Design review of the part built by this model. Coordinates are the model's own, in mm. Face numbers are marked on the shaded views. A direction names the side the tool comes from. Coordinates: 2 decimals unless noted, no trailing zeros. Write each loop counter-clockwise with the first axis right and the second up, starting at its lowest first coordinate (ties: lowest second). Pieces come first, ordered by that corner, then holes. Notation, with made-up numbers: (1, -13) -> (29, -13) arc R18 cw to (29, -7) -> close; hole circle Ø8 at (15.5, 87.25). An arc over 180 degrees is marked (long way). Return JSON: item names as keys, results as strings. Group by question number.
from build123d import *

# Parameters (mm, degrees)
F1_DEPTH = 5
F2_W     = 30
F2_H     = 5
F3_DEPTH = 5
F5_DEPTH = 5.001


with BuildPart() as f1:
    # F0 (on Top) → F1 (new body)
    with BuildSketch(Plane.XY):
        Polygon((-35, -80), (35, -80), (-35, -15.451086), align=None)
    extrude(amount=F1_DEPTH)

    # F2 (on face) → F3 (join)
    with BuildSketch(Plane.XY.offset(5)):
        with Locations((15, -82.5)):
            Rectangle(F2_W, F2_H)
    extrude(amount=-F3_DEPTH)

    # F4 (on face) → F5 (cut, through all)
    with BuildSketch(Plane.XY.offset(5)):
        with BuildLine():
            Line((-24.877707, -45.415195), (-23.765102, -50.289835))
            Line((-23.765102, -50.289835), (-26.882551, -54.198992))
            ThreePointArc((-26.882551, -54.198992), (-25.495156, -55.938731), (-25, -58.10815))
            ThreePointArc((-25, -58.10815), (-25.110116, -59.151716), (-25.435612, -60.149317))
            ThreePointArc((-25.435612, -60.149317), (-17.311619, -57.928719), (-13.765102, -50.289835))
            ThreePointArc((-13.765102, -50.289835), (-15.773609, -44.278509), (-20.992311, -40.681941))
            ThreePointArc((-20.992311, -40.681941), (-22.125625, -43.712968), (-24.877707, -45.415195))
        make_face()
        with BuildLine():
            Line((-26.882551, -54.198992), (-23.765102, -50.289835))
            Line((-23.765102, -50.289835), (-24.877707, -45.415195))
            ThreePointArc((-24.877707, -45.415195), (-28.095815, -45.075625), (-30.43201, -42.836491))
            ThreePointArc((-30.43201, -42.836491), (-33.514381, -48.064626), (-33.005663, -54.112403))
            ThreePointArc((-33.005663, -54.112403), (-29.9293, -53.10865), (-26.882551, -54.198992))
        make_face()
    extrude(amount=-F5_DEPTH, mode=Mode.SUBTRACT)


solid = f1.part
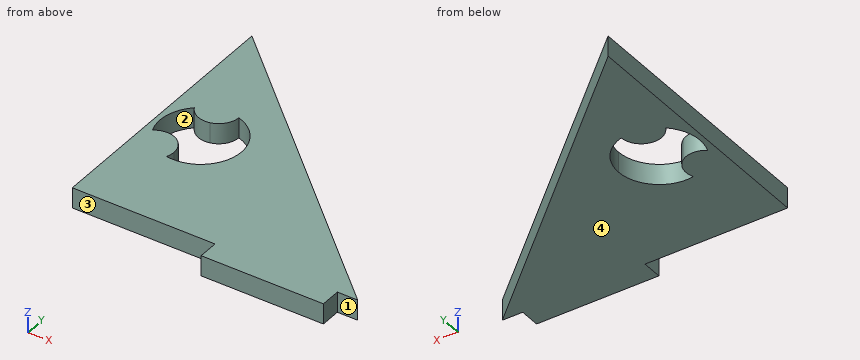
Q1. We need section C-C on x = -23. Write out the cut boundary in (y, z).
Q2. For P1, Ø2, axis at x = -16.5, z = 4, coming from the -Y side; P2, Ø1, axis at x = 0.5, z = 4.5, coming from the +Y side; P3, Ø2.5, axis at y = -82, z = 3.5, coming from the -X side, all flat-tipped, find the tip position at first contact; note any pin that passes through.
Q3. We need section D-D on y = -66.5. Write out the cut boundary in (x, z), plus the area to 3 significant figures.
Q4. For the marked faces 3 and 4, list the 3-axis set-ups (+Z, -Z, +X, -X, +Y, -Y) from which the entire face can be reached by the end or side of a thin tool; tool diameter is ignored.
Q5. We need section A-A on y = -49. Write out the cut boundary in (x, z), plus the area to 3 significant figures.
Q6. The part is to be moulded in two halves that separate along X. For the marked faces 1 and 2, say which applies: +X half, -X half, draft (parallel to the pull), parting line (faces both ways), or undercut.
Q7. Wall thickness on L1, parallel to X at y = -54, z = 0.9; L2, parallel to X at y = -81.5, z = 3.05; L3, parallel to X at y = -53.5, z = 4: over which ranges is each line inside the solid? List them lowest first.
Q8. We need section B-B on z = 1.3. Write out the cut boundary in (x, y), plus the area to 3 significant figures.
Findings below:
{
 "1": {"outline": "(-80, 0) -> (-60.26, 0) -> (-60.26, 5) -> (-80, 5) -> close; (-44.55, 0) -> (-26.52, 0) -> (-26.52, 5) -> (-44.55, 5) -> close"},
 "2": {"P1": "stops at y = -80", "P2": "stops at y = -47.73", "P3": "stops at x = 0"},
 "3": {"outline": "(-35, 0) -> (20.36, 0) -> (20.36, 5) -> (-35, 5) -> close", "area": "277 mm^2"},
 "4": {"face 3": "+Z, -Z, -X, -Y", "face 4": "-Z, +X, -X, +Y, -Y"},
 "5": {"outline": "(-35, 0) -> (-33.68, 0) -> (-33.68, 5) -> (-35, 5) -> close; (-13.85, 0) -> (1.38, 0) -> (1.38, 5) -> (-13.85, 5) -> close", "area": "82.7 mm^2"},
 "6": {"face 1": "draft", "face 2": "undercut"},
 "7": {"L1": "x = -35 to -33.05, -32.85 to -27.15, -14.48 to 6.8", "L2": "x = 0 to 30", "L3": "x = -35 to -33.24, -31.94 to -28.06, -14.29 to 6.26"},
 "8": {"outline": "(-35, -80) -> (0, -80) -> (0, -85) -> (30, -85) -> (30, -80) -> (35, -80) -> (-35, -15.45) -> close; hole (-33.01, -54.11) arc R5 cw to (-26.88, -54.2) arc R5 cw to (-25, -58.11) arc R5 cw to (-25.44, -60.15) arc R10 ccw to (-20.99, -40.68) arc R5 cw to (-24.88, -45.42) arc R5 cw to (-30.43, -42.84) arc R10 ccw to start", "area": "2,170 mm^2"}
}
